For this review, use the dimensioned drawing (mm, ordinates from the lowest corner) and the shaded views. A direction names the side the tool comes from. Coordinates: 2 decimals unless noted, no trailing zeros. Order: outer loops, then holes, each group sorted by start corner. A loop starts at its lowest first (then second) coordinate and runs counter-clockwise, first axis right, second up. Notation, with made-up numbers: M 56,89 L 67,89 A11 ccw 67,109 Z; hole C -5,34.5 d5. An arc over 180 degrees is marked long. Answer in a Markdown table with one row per item.
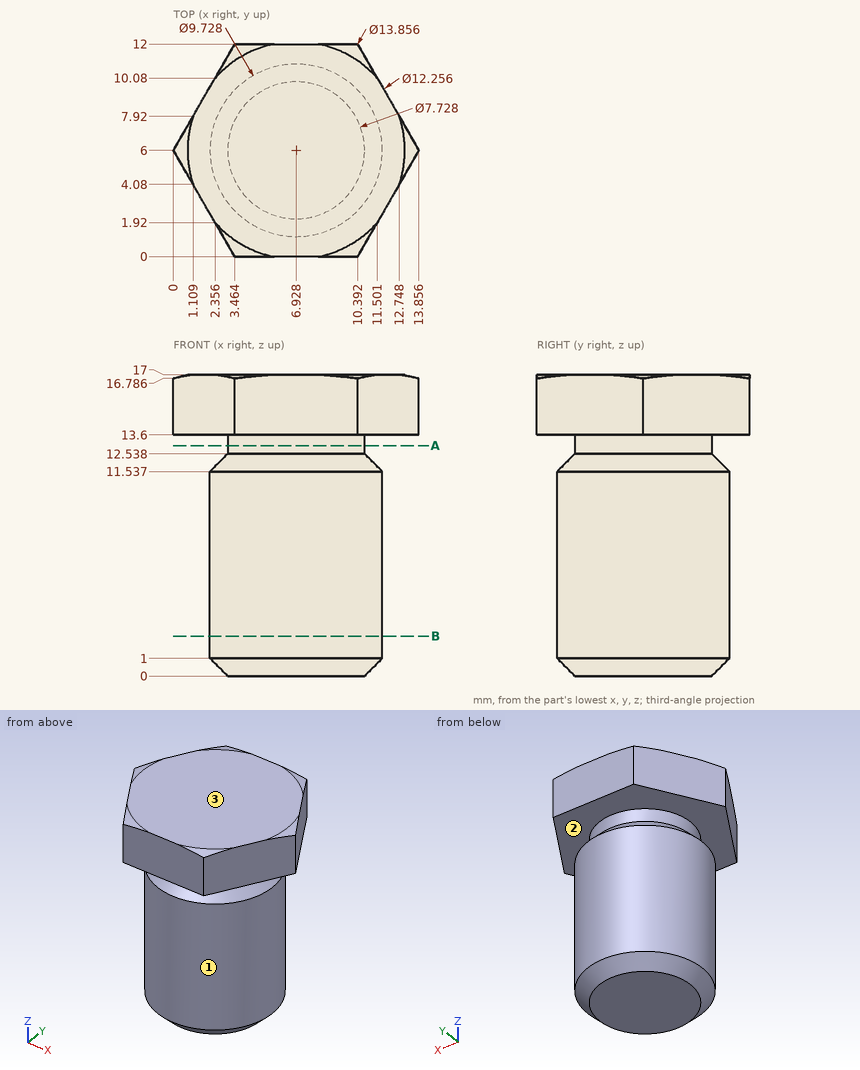
(1) For the marked faces 1, 2 and 3, list the 3-axis set-ups (+Z, -Z, +X, -X, +Y, -Y) from which the entire face can be reached by the end or side of a thin tool; tool diameter is ignored.
Return value:
| item | result |
|---|---|
| face 1 | -Z |
| face 2 | none |
| face 3 | +Z, +X, -X, +Y, -Y |
(2) Insertion check: pin 1 Ø5 at (x, z) = (9, 3) entering from +Y; pin 2 Ø1 at (x, z) = (7, 7.5) entering from -Y; pin 3 Ø2 at (y, z) = (6.5, 8.5) entering from +X. Each pin has a flat end and moves straight along its axis. Give the tip position at first contact, or say it passes through.
Return value:
| item | result |
|---|---|
| pin 1 | stops at y = 10.86 |
| pin 2 | stops at y = 1.14 |
| pin 3 | stops at x = 11.79 |
(3) Add section A-A, the plane z = 13. Give the boundary of the cut face in (x, y) (1 decimal).
Return value:
| item | result |
|---|---|
| outline | C 6.9,6 d7.7 |
(4) Add section B-B, the plane z = 2.25. Give the boundary of the cut face in (x, y) (1 decimal).
Return value:
| item | result |
|---|---|
| outline | C 6.9,6 d9.7 |
(5) For line 1 along Z through (x, y) = (4, 10.75); line 2 along Z through (x, y) = (9.75, 9.25) (1 decimal); line 3 along Y through (x, z) = (7, 3.25), list the stretches that pass through material, from the lowest coordinate up. Write a range as from..to.
Return value:
| item | result |
|---|---|
| line 1 | z = 13.6..17 |
| line 2 | z = 0.4..12.1, 13.6..17 |
| line 3 | y = 1.14..10.86 |
